from build123d import *

# Parameters (mm, degrees)
SKETCH_1_R      = 1.5
EXTRUDE_1_DEPTH = 20
EXTRUDE_START   = 2.5
SKETCH_2_R      = 2
SKETCH_2_R_2    = 1.5
EXTRUDE_2_DEPTH = 0.4
FILLET_1_R      = 0.1


with BuildPart() as part:
    # 草图1 → 凸台-拉伸1 (new body)
    with BuildSketch(Plane(origin=(0, 0, 0), x_dir=(1, 0, 0), z_dir=(0, 1, 0))):
        with Locations(Location((0, 0, 0), (0, 0, 270))):
            Circle(SKETCH_1_R)
    extrude(amount=EXTRUDE_1_DEPTH)

    # 草图2 → 凸台-拉伸2 (add)
    with BuildSketch(Plane.XZ.offset(-20).offset(EXTRUDE_START)):
        with Locations(Location((0, 0, 0), (0, 0, 270))):
            Circle(SKETCH_2_R)
        with Locations(Location((0, 0, 0), (0, 0, 270))):
            Circle(SKETCH_2_R_2, mode=Mode.SUBTRACT)
    extrude(amount=-EXTRUDE_2_DEPTH)

    # 圆角1
    fillet_1_edges = [part.edges().sort_by_distance(p)[0] for p in [
        (0, 0, -1.5),
        (0, 20, -1.5),
        (0, 17.5, 2),
        (0, 17.9, 2),
    ]]
    fillet(fillet_1_edges, radius=FILLET_1_R)


solid = part.part
The model under review builds one solid part; all positions refer to its coordinate system, in mm. A direction names the side the tool comes from. Round coordinates to 2 decimals unless told otherwise and drop trailing zeros. Order: outer loops, then holes, each group sorted by start corner. A loop starts at its lowest first (then second) coordinate and runs counter-clockwise, first axis right, second up. Notation, with made-up numbers: (-2, -8) -> (31, -8) arc R34 cw to (31, 24) -> close; hole circle Ø7 at (32.5, 34.5). An arc over 180 degrees is marked (long way). Write item = value, one per line. Start each with the question number.
Item 1: Consider section C-C on y = 4.5. Write out the cut boundary in (x, z), plus the area to 3 significant figures.
Item 2: For faces 1 (the face through (0.45, 18.89, 1.43)), 2 (the face through (0.45, 8.68, 1.43)), 3 (the face through (0, 0, 0)), list the 3-axis set-ups (+Z, -Z, +X, -X, +Y, -Y) from which the entire face can be reached by the end or side of a thin tool; tool diameter is ignored.
Item 3: Clearance check with flat-ended pins moving along their axes: pin 1 Ø1.5 at (y, z) = (14.5, 0.5) entering from -X; pin 2 Ø1.5 at (x, z) = (-0.5, 1.5) entering from +Y; pin 3 Ø1 at (y, z) = (4, 0) entering from +X. State where each tip first meets the part, or that it passes through.
Item 4: For line 1 along X through (y, z) = (3.75, 0); line 2 along Y through (x, z) = (1.7, 0), list the stretches that pass through material, from the lowest coordinate up.
Item 5: Consider section B-B on z = 0. Write out the cut boundary in (x, y).
Item 6: Consider section A-A on x = 0. Write out the cut boundary in (y, z).
Conclusion:
q1.outline = circle Ø3 at (0, 0)
q1.area = 7.07 mm2
q2.face_1 = +Y
q2.face_2 = -Y
q2.face_3 = +Z, -Z, +X, -X, -Y
q3.pin_1 = -1.5
q3.pin_2 = 20
q3.pin_3 = 1.5
q4.line_1 = -1.5 to 1.5
q4.line_2 = 17.5 to 17.9
q5.outline = (-2, 17.6) arc R0.1 ccw to (-1.9, 17.5) -> (-1.5, 17.5) -> (-1.5, 0.1) arc R0.1 ccw to (-1.4, 0) -> (1.4, 0) arc R0.1 ccw to (1.5, 0.1) -> (1.5, 17.5) -> (1.9, 17.5) arc R0.1 ccw to (2, 17.6) -> (2, 17.8) arc R0.1 ccw to (1.9, 17.9) -> (1.5, 17.9) -> (1.5, 19.9) arc R0.1 ccw to (1.4, 20) -> (-1.4, 20) arc R0.1 ccw to (-1.5, 19.9) -> (-1.5, 17.9) -> (-1.9, 17.9) arc R0.1 ccw to (-2, 17.8) -> close
q6.outline = (0, -1.4) arc R0.1 ccw to (0.1, -1.5) -> (17.5, -1.5) -> (17.5, -1.9) arc R0.1 ccw to (17.6, -2) -> (17.8, -2) arc R0.1 ccw to (17.9, -1.9) -> (17.9, -1.5) -> (19.9, -1.5) arc R0.1 ccw to (20, -1.4) -> (20, 1.4) arc R0.1 ccw to (19.9, 1.5) -> (17.9, 1.5) -> (17.9, 1.9) arc R0.1 ccw to (17.8, 2) -> (17.6, 2) arc R0.1 ccw to (17.5, 1.9) -> (17.5, 1.5) -> (0.1, 1.5) arc R0.1 ccw to (0, 1.4) -> close
